Can you work these out from the model? Positions are in its coordinate system, mm. Face numbers are marked on the shaded views. A direction names the side the tool comes from. Give positions to 0.01 mm unless a question says otherwise; leave off trailing zeros. Loops run counter-clockwise (first coordinate to the right, second up) from the corner with the lowest first, then second, coordinate; pieces in that order, holes last. Notation, with made-up numbers: (21, 52.25) - (72, 52.25) arc R16 cw to (72, 62.25) - close; hole circle Ø3 at (28, 55.5). An arc over 180 degrees is marked (long way). Answer as a JSON object with one key per item and string values.
```python
from build123d import *

# Parameters (mm, degrees)
SKETCH1_R           = 3
BOSS_EXTRUDE1_DEPTH = 10
SKETCH2_R           = 2.45
BOSS_EXTRUDE2_DEPTH = 0.65
SKETCH3_R           = 3
BOSS_EXTRUDE3_DEPTH = 8.67
BOSS_EXTRUDE4_DEPTH = 5
SKETCH5_R           = 3
BOSS_EXTRUDE5_DEPTH = 20.5


with BuildPart() as part:
    # Sketch1 → Boss-Extrude1 (new body)
    with BuildSketch(Plane(origin=(0, 0, 0), x_dir=(1, 0, 0), z_dir=(0, 1, 0))):
        with Locations(Location((0, 0, 0), (0, 0, 270))):
            Circle(SKETCH1_R)
    extrude(amount=BOSS_EXTRUDE1_DEPTH)

    # Sketch2 → Boss-Extrude2 (add)
    with BuildSketch(Plane(origin=(0, 10, 0), x_dir=(1, 0, 0), z_dir=(0, 1, 0))):
        with Locations(Location((0, 0, 0), (0, 0, 270))):
            Circle(SKETCH2_R)
    extrude(amount=BOSS_EXTRUDE2_DEPTH)

    # Sketch3 → Boss-Extrude3 (add)
    with BuildSketch(Plane(origin=(0, 10.65, 0), x_dir=(1, 0, 0), z_dir=(0, 1, 0))):
        with Locations(Location((0, 0, 0), (0, 0, 270))):
            Circle(SKETCH3_R)
    extrude(amount=BOSS_EXTRUDE3_DEPTH)

    # Sketch4 → Boss-Extrude4 (add)
    with BuildSketch(Plane(origin=(0, 19.32, 0), x_dir=(1, 0, 0), z_dir=(0, 1, 0))):
        with BuildLine():
            Line((-2, -2), (2.236067977, -2))
            ThreePointArc((2.236067977, -2), (2.802517077, -1.070466269), (3, 0))
            ThreePointArc((3, 0), (2.121320344, 2.121320344), (0, 3))
            ThreePointArc((0, 3), (-1.070466269, 2.802517077), (-2, 2.236067977))
            Line((-2, 2.236067977), (-2, -2))
        make_face()
    extrude(amount=BOSS_EXTRUDE4_DEPTH)

    # Sketch5 → Boss-Extrude5 (add)
    with BuildSketch(Plane(origin=(0, 24.32, 0), x_dir=(1, 0, 0), z_dir=(0, 1, 0))):
        with Locations(Location((0, 0, 0), (0, 0, 270))):
            Circle(SKETCH5_R)
    extrude(amount=BOSS_EXTRUDE5_DEPTH)


solid = part.part
```
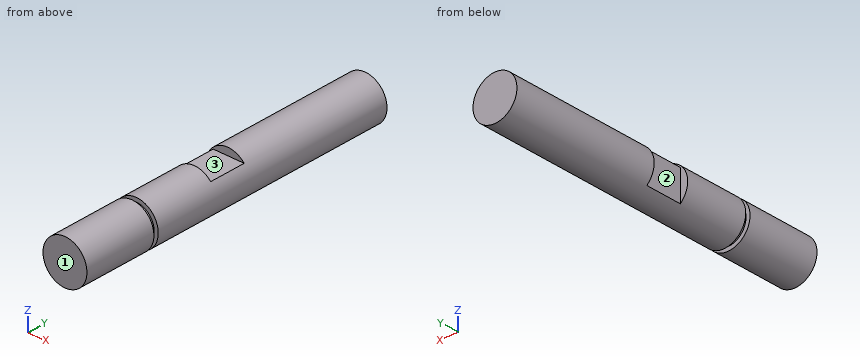
1) Imagine slicing it at B-B on x = 0. Write out the boundary of the cut face in (y, z), and give its area (3 significant figures).
Check sheet entries:
{"outline": "(0, -3) - (10, -3) - (10, -2.45) - (10.65, -2.45) - (10.65, -3) - (44.82, -3) - (44.82, 3) - (24.32, 3) - (24.32, 2) - (19.32, 2) - (19.32, 3) - (10.65, 3) - (10.65, 2.45) - (10, 2.45) - (10, 3) - (0, 3) - close", "area": "263 mm2"}
2) I need wall thicknesses on L1, parallel to Y at x = -0.5, z = -2.6; L2, parallel to Z at x = 2, y = 35.5; L3, parallel to Z at x = 0.2, y = 39. Which ranges of each line are inside material? Lowest first, please.
Check sheet entries:
{"L1": "0 to 10, 10.65 to 44.82", "L2": "-2.24 to 2.24", "L3": "-2.99 to 2.99"}
3) Imagine slicing it at C-C on y = 33. Write out the boundary of the cut face in (x, z).
Check sheet entries:
{"outline": "circle Ø6 at (0, 0)"}
4) Imagine slicing it at A-A on z = 0.95. Write out the boundary of the cut face in (x, y).
Check sheet entries:
{"outline": "(-2.85, 0) - (2.85, 0) - (2.85, 10) - (2.26, 10) - (2.26, 10.65) - (2.85, 10.65) - (2.85, 44.82) - (-2.85, 44.82) - (-2.85, 24.32) - (-2, 24.32) - (-2, 19.32) - (-2.85, 19.32) - (-2.85, 10.65) - (-2.26, 10.65) - (-2.26, 10) - (-2.85, 10) - close"}
5) I'm going to push flat-ended pins straight in: P1, Ø1.5, axis at y = 31, z = -1.5, coming from the +X side; P2, Ø1.3, axis at y = 21, z = 0, coming from the -X side; P3, Ø1, axis at y = 26.5, z = 1.5, coming from the +X side. Where does each tip first touch, or does it pass through?
Check sheet entries:
{"P1": "x = 2.9", "P2": "x = -2", "P3": "x = 2.83"}
6) Which directions (+Z, -Z, +X, -X, +Y, -Y) give clear straight access to the entire face, cutting with the end or side of a thin tool? Please do the marked faces 1, 2 and 3.
Check sheet entries:
{"face 1": "+Z, -Z, +X, -X, -Y", "face 2": "+Z, -Z, -X", "face 3": "+Z, +X, -X"}
